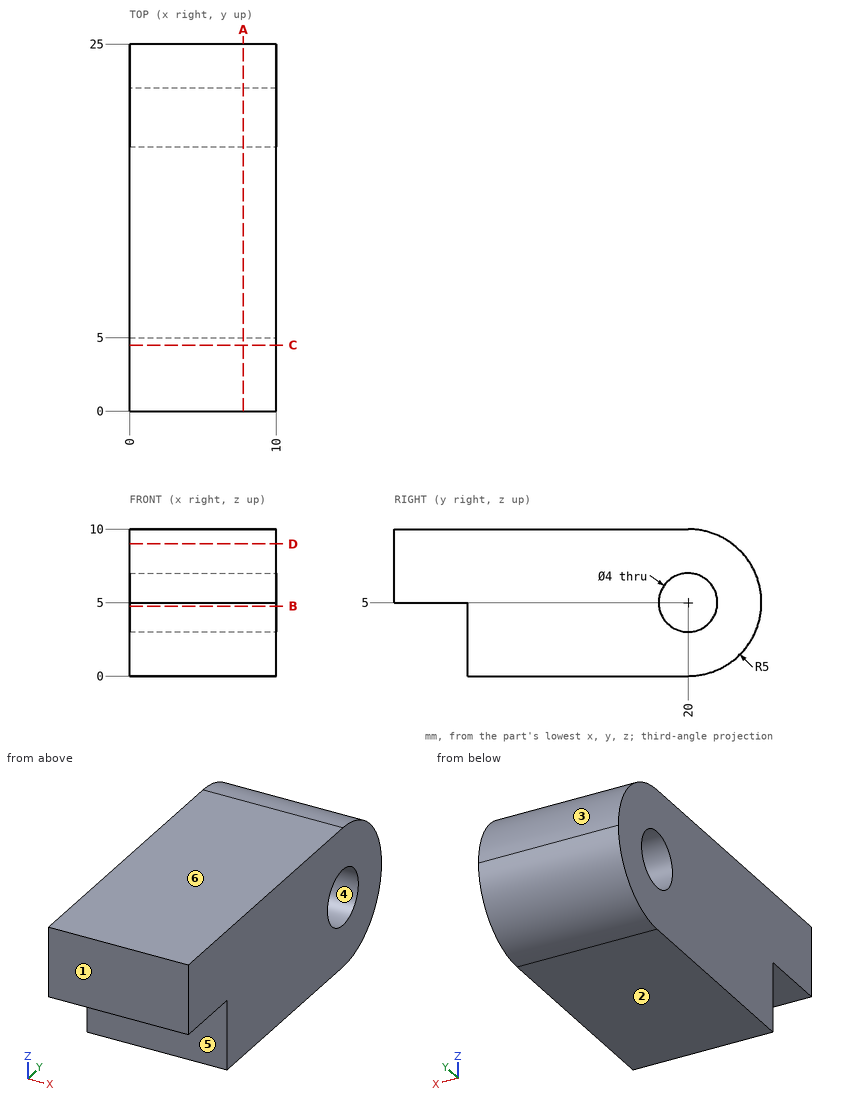
Source: three-view drawing plus pictorial views. Frame: mm from the lowest corner of the part. A direction names the side the tool comes from. Round coordinates to 2 decimals unless told otherwise and drop trailing zeros. Loops run counter-clockwise (first coordinate to the right, second up) from the corner with the lowest first, then second, coordinate; pieces in that order, holes last.
Item 1: Reachability of the marked faces 5 and 6 from +Z, -Z, +X, -X, +Y, -Y: full face, straight path, thin tool, end or side. Return the list, or none.
Checked values:
face 5: -Z, +X, -X, -Y
face 6: +Z, +X, -X, +Y, -Y
Item 2: Contact query for flat-ended pins moving along their axis: P1, Ø2, axis at x = 2.5, z = 2, coming from the -Y side; P2, Ø1, axis at x = 2, z = 6.5, coming from the +Y side. Output: stop coordinate, or through.
Checked values:
P1: stops at y = 5
P2: stops at y = 24.9
Item 3: Section B-B, the plane z = 4.75. Output: boundary loops of the cut face in (x, y).
Checked values:
outline: (0, 5) - (10, 5) - (10, 18.02) - (0, 18.02) - close; (0, 21.98) - (10, 21.98) - (10, 24.99) - (0, 24.99) - close
Item 4: Mould query, pull axis Y, two halves, no side actions, for the marked faces 1, 2, 3 and 4. Classes: released by +Y, released by -Y, zero draft, split by the parting line, or undercut.
Checked values:
face 1: released by -Y
face 2: zero draft
face 3: released by +Y
face 4: undercut
Item 5: Section C-C, the plane y = 4.5. Output: boundary loops of the cut face in (x, z).
Checked values:
outline: (0, 5) - (10, 5) - (10, 10) - (0, 10) - close
Item 6: Section A-A, the plane x = 7.75. Output: boundary loops of the cut face in (y, z).
Checked values:
outline: (0, 5) - (5, 5) - (5, 0) - (20, 0) arc R5 ccw to (25, 5) arc R5 ccw to (20, 10) - (0, 10) - close; hole circle Ø4 at (20, 5)
Item 7: Line query: L1, parallel to Z at x = 6.5, y = 20; L2, parallel to Z at x = 8, y = 20.5 (1 decimal); L3, parallel to Z at x = 7.5, y = 2.5. Output: solid intervals per line, ascending.
Checked values:
L1: z = 0 to 3, 7 to 10
L2: z = 0 to 3.1, 6.9 to 10
L3: z = 5 to 10
Item 8: Section D-D, the plane z = 9. Output: boundary loops of the cut face in (x, y), plus the area to 3 significant figures.
Checked values:
outline: (0, 0) - (10, 0) - (10, 23) - (0, 23) - close
area: 230 mm2
